```python
from build123d import *

# Parameters (mm, degrees)
SKETCH1_R           = 5
SKETCH1_R_2         = 4
BOSS_EXTRUDE1_DEPTH = 3
FILLET1_R           = 100
SKETCH2_R           = 2
CUT_EXTRUDE1_DEPTH  = 3
FILLET2_R           = 2


with BuildPart() as part:
    # Sketch1 → Boss-Extrude1 (new body)
    with BuildSketch(Plane(origin=(0, 0, 0), x_dir=(1, 0, 0), z_dir=(0, 1, 0))):
        with BuildLine():
            Line((0, 15), (-96.417851723, 41.525419301))
            Line((-96.417851723, 41.525419301), (-302.012777379, 24.918842815))
            ThreePointArc((-302.012777379, 24.918842815), (-323.422288966, -8.74050225), (-285.196078396, -20.145567878))
            Line((-285.196078396, -20.145567878), (-244.853395733, 9.500154448))
            Line((-244.853395733, 9.500154448), (-94.853395733, 15.263592787))
            Line((-94.853395733, 15.263592787), (-8.209432186, -12.55409189))
            Line((-8.209432186, -12.55409189), (0, -15))
            Line((0, -15), (35, -15))
            ThreePointArc((35, -15), (50, 0), (35, 15))
            Line((35, 15), (0, 15))
        make_face()
        with Locations(Location((0, 0, 0), (0, 0, 270))):
            Circle(SKETCH1_R, mode=Mode.SUBTRACT)
        with Locations(Location((35, 0, 0), (0, 0, 270))):
            Circle(SKETCH1_R_2, mode=Mode.SUBTRACT)
    extrude(amount=BOSS_EXTRUDE1_DEPTH)

    # Fillet1
    fillet1_edges = [part.edges().sort_by_distance(p)[0] for p in [
        (0, 1.5, -15),
        (-96.417851723, 1.5, -41.525419301),
        (-94.853395733, 1.5, -15.263592787),
        (-244.853395733, 1.5, -9.500154448),
        (0, 1.5, 15),
    ]]
    fillet(fillet1_edges, radius=FILLET1_R)

    # Sketch2 → Cut-Extrude1 (cut)
    with BuildSketch(Plane(origin=(0, 3, 0), x_dir=(1, 0, 0), z_dir=(0, 1, 0))):
        with Locations(Location((-100.410325029, 29.966674425, 0), (0, 0, 270))):
            Circle(SKETCH2_R)
        with Locations(Location((-154.331360865, 23.327852047, 0), (0, 0, 270))):
            Circle(SKETCH2_R)
        with Locations(Location((-194.43609766, 21.998076888, 0), (0, 0, 270))):
            Circle(SKETCH2_R)
        with Locations(Location((-250.479012244, 9.089087069, 0), (0, 0, 270))):
            Circle(SKETCH2_R)
        with Locations(Location((-305.880435037, 12.401187858, 0), (0, 0, 270))):
            Circle(SKETCH2_R)
        with Locations(Location((-295.391832737, -15.705559051, 0), (0, 0, 270))):
            Circle(SKETCH2_R)
        Polygon((-292.21586201, 18.687373798), (-281.876511166, -9.019417731), (-238.23936591, 23.047232428), align=None)
        Polygon((-17.754718765, 16.773026019), (-17.754718765, -6.33868172), (-53.365436428, 5.0944023), align=None)
        Polygon((-22.990022437, 18.213305206), (-69.89582428, 31.117513703), (-58.230092835, 6.656236183), align=None)
        Polygon((-62.154702225, 7.916261025), (-73.721446188, 32.169976742), (-92.622909187, 17.698303988), align=None)
        Polygon((-77.35185331, 33.168734435), (-96.92030532, 18.186389746), (-96.703582242, 38.492569336), align=None)
        Polygon((-244.106325436, 12.531072737), (-222.617491874, 28.322089864), (-214.487999018, 13.66909539), align=None)
        Polygon((-106.555479442, 37.696799286), (-100.410325029, 18.05229299), (-131.520316701, 16.856956198), align=None)
        Polygon((-111.738383291, 37.278159142), (-136.427588937, 16.668404458), (-141.03422906, 34.911837591), align=None)
        Polygon((-144.066545636, 34.666907435), (-139.492021115, 16.550660019), (-153.569970314, 16.009744071), align=None)
        Polygon((-153.429835368, 33.910603812), (-162.727242525, 15.657894913), (-172.020743917, 32.408955151), align=None)
        Polygon((-175.304372068, 32.143725735), (-166.086412512, 15.528825786), (-197.65154914, 14.316000995), align=None)
        Polygon((-219.333863723, 28.58731928), (-211.128829032, 13.798164517), (-189.577714365, 30.990821062), align=None)
    extrude(amount=-CUT_EXTRUDE1_DEPTH, mode=Mode.SUBTRACT)

    # Fillet2
    fillet2_edges = [part.edges().sort_by_distance(p)[0] for p in [
        (-96.92030532, 1.5, -18.186389746),
        (-96.703582242, 1.5, -38.492569336),
        (-77.35185331, 1.5, -33.168734435),
        (-17.754718765, 1.5, -16.773026019),
        (-17.754718765, 1.5, 6.33868172),
        (-22.990022437, 1.5, -18.213305206),
        (-58.230092835, 1.5, -6.656236183),
        (-69.89582428, 1.5, -31.117513703),
        (-62.154702225, 1.5, -7.916261025),
        (-92.622909187, 1.5, -17.698303988),
        (-73.721446188, 1.5, -32.169976742),
        (-214.487999018, 1.5, -13.66909539),
        (-244.106325436, 1.5, -12.531072737),
        (-222.617491874, 1.5, -28.322089864),
        (-219.333863723, 1.5, -28.58731928),
        (-189.577714365, 1.5, -30.990821062),
        (-211.128829032, 1.5, -13.798164517),
        (-172.020743917, 1.5, -32.408955151),
        (-153.429835368, 1.5, -33.910603812),
        (-162.727242525, 1.5, -15.657894913),
        (-141.03422906, 1.5, -34.911837591),
        (-111.738383291, 1.5, -37.278159142),
        (-136.427588937, 1.5, -16.668404458),
        (-131.520316701, 1.5, -16.856956198),
        (-106.555479442, 1.5, -37.696799286),
        (-100.410325029, 1.5, -18.05229299),
        (-153.569970314, 1.5, -16.009744071),
        (-144.066545636, 1.5, -34.666907435),
        (-139.492021115, 1.5, -16.550660019),
        (-197.65154914, 1.5, -14.316000995),
        (-175.304372068, 1.5, -32.143725735),
        (-166.086412512, 1.5, -15.528825786),
        (-292.21586201, 1.5, -18.687373798),
        (-238.23936591, 1.5, -23.047232428),
        (-281.876511166, 1.5, 9.019417731),
    ]]
    fillet(fillet2_edges, radius=FILLET2_R)


solid = part.part
```
The model under review builds one solid part; all positions refer to its coordinate system, in mm. A direction names the side the tool comes from. Give positions to 0.01 mm unless a question says otherwise; leave off trailing zeros. Write each loop counter-clockwise with the first axis right and the second up, starting at its lowest first coordinate (ties: lowest second). Pieces come first, ordered by that corner, then holes.
(1) Tool access review of faces 1 (the flat face through (-231.75, 1.52, -21.61)), 2 (the flat face through (-277.495, 1.479, 14.486)): name each direction out of +Z, -Z, +X, -X, +Y, -Y from which nothing blocks a thin tool from reaching the whole face with its end or side.
(2) For P1, Ø3, axis at x = -295.39, z = 15.71, coming from the +Y side; P2, Ø1.5, axis at x = 20.5, y = 2, coming from the -Z side, all flat-tipped, find the tip position at first contact; note any pin that passes through.
(3) Consider section B-B, the plane y = 1.2. Give the number of separate pieces and of enclosed holes in the cut face, and give its area (3 significant figures).
(4) Consider section A-A, the plane x = -85. Give the boundary of the cut face in (y, z).
(5) The part is to be moulded in two halves that separate along X. For faces 3 (the flat face through (-87.013, 1.521, -25.772)), 4 (the cylindrical face through (50, 1, 0)), say which applies: released by +X, released by -X, zero draft, split by the parting line, or undercut.
(6) To check wall thickness, follow L1, parallel to Z at x = -170, y = 1.5; L2, parallel to Z at x = -92.5, y = 2.35; L3, parallel to Z at x = -50, y = 1.95. State the ranges of each line that lie inside material, in increasing order.
Returned:
1. face 1: +Y, -Y
1. face 2: +Z, +Y, -Y
2. P1: passes through
2. P2: stops at z = -15
3. separate pieces: 1
3. enclosed holes: 20
3. area: 6,810 mm2
4. outline: (0, -38.21) - (3, -38.21) - (3, -35.27) - (0, -35.27) - close; (0, -27.31) - (3, -27.31) - (3, -23.53) - (0, -23.53) - close; (0, -15.25) - (3, -15.25) - (3, -11.83) - (0, -11.83) - close
5. face 3: undercut
5. face 4: released by +X
6. L1: z = -35.58 to -32.24, -28.77 to -22.58, -15.38 to -12.38
6. L2: z = -39.52 to -37.34, -21.57 to -13.35
6. L3: z = -28.76 to -25.64, -9.36 to -6.2, -4.01 to -0.86
